The model under review builds one solid part; all positions refer to its coordinate system, in mm. Face numbers are marked on the shaded views. A direction names the side the tool comes from. Give positions to 0.01 mm unless a question says otherwise; leave off trailing zeros. Loops run counter-clockwise (first coordinate to the right, second up) from the corner with the lowest first, then second, coordinate; pieces in that order, holes last. Notation, with made-up numbers: (23, 54.5) -> (38, 54.5) arc R21 cw to (38, 88.5) -> close; hole circle Ø4 at (12, 70). An arc over 180 degrees is marked (long way). Write each question's results on one line, items separated by ' | '. Start each with the question number.
Q1. Mouldability with a two-part tool opening along Y and no side actions: class the marked faces 1, 2 and 3 as released by +Y, released by -Y, zero draft, split by the parting line, or undercut.
Q2. Wall thickness on L1, parallel to X at y = 2.95, z = 108.5; L2, parallel to X at y = 3, z = 120; L3, parallel to Y at x = 35, z = 66: over which ranges is each line inside the solid? List them lowest first. Write a range as [from, to].
Q3. Insertion check: pin 1 Ø4 at (x, z) = (27.5, 82) entering from +Y; pin 2 Ø2.5 at (y, z) = (3.5, 99) entering from -X; pin 3 Ø1.5 at (y, z) = (1.5, 98.5) entering from +X. Each pin has a flat end and moves straight along its axis. Give the tip position at first contact, or say it passes through.
Q4. We need section C-C (x = 3.5). Write out the cut boundary in (y, z), plus the area to 3 significant figures.
Q5. We need section B-B (y = 17.5). Write out the cut boundary in (x, z).
Q6. Machinability: for the marked faces 4 and 5, which of the approach directions +Z, -Z, +X, -X, +Y, -Y give a long, thin tool a straight path to every point of the face, cutting with its end or side? Answer none if there is none.
Q7. We need section A-A (z = -42). Write out the cut boundary in (x, y), plus the area to 3 significant figures.
Q8. We need section D-D (z = 72.5). Write out the cut boundary in (x, y), plus the area to 3 significant figures.
from build123d import *

# Parameters (mm, degrees)
SCHIZZO2_W                   = 15
SCHIZZO2_H                   = 5
SCHIZZO5_W                   = 15
SCHIZZO5_H                   = 5
SCHIZZO9_R                   = 3
SCHIZZO9_R_2                 = 4
ESTRUSIONE_ESTRUSIONE1_DEPTH = 5
SCHIZZO10_R                  = 3
TAGLIO_ESTRUSIONE1_DEPTH     = 144.674980425


with BuildPart() as part:
    # Sweep1: sweep along a path in Schizzo1
    with BuildLine(Plane.ZY) as sweep1_path:
        Line((0, 0), (-80, 0))
        ThreePointArc((-80, 0), (-97.5, 17.5), (-80, 35))
        Line((-80, 35), (-20, 35))
        ThreePointArc((-20, 35), (-4.629573851, 25.866600265), (-5.303061543, 8))
    # Schizzo2 → Sweep1 (sweep)
    with BuildSketch(Plane(origin=(0, 0, 0), x_dir=(-1, 0, 0), z_dir=(0, 0, -1))):
        with Locations((0, 2.5)):
            Rectangle(SCHIZZO2_W, SCHIZZO2_H)
    sweep(path=sweep1_path.line)

    # Sweep2: sweep along a path in Schizzo3
    with BuildLine(Plane.XZ) as sweep2_path:
        ThreePointArc((42.5, 96.5), (37.98987096, 70.837222968), (25, 48.25))
        ThreePointArc((25, 48.25), (12.01012904, 25.662777032), (7.5, 0))
    # Schizzo5 → Sweep2 (sweep)
    with BuildSketch(Plane.XY):
        with Locations((0, 2.5)):
            Rectangle(SCHIZZO5_W, SCHIZZO5_H)
    sweep(path=sweep2_path.line)

    # Schizzo9 → Estrusione-Estrusione1 (add)
    with BuildSketch(Plane.XZ):
        with BuildLine():
            Line((25, 96.5), (45, 96.5))
            Line((45, 96.5), (45, 102.126136458))
            ThreePointArc((45, 102.126136458), (49.5, 109), (45, 115.873863542))
            Line((45, 115.873863542), (45, 121.5))
            ThreePointArc((45, 121.5), (35, 131.5), (25, 121.5))
            Line((25, 121.5), (25, 115.873863542))
            ThreePointArc((25, 115.873863542), (20.5, 109), (25, 102.126136458))
            Line((25, 102.126136458), (25, 96.5))
        make_face()
        with Locations(Location((35, 120.5, 0), (0, 0, 270))):
            Circle(SCHIZZO9_R, mode=Mode.SUBTRACT)
        with Locations(Location((35, 108.5, 0), (0, 0, 270))):
            Circle(SCHIZZO9_R_2, mode=Mode.SUBTRACT)
    extrude(amount=-ESTRUSIONE_ESTRUSIONE1_DEPTH)

    # Schizzo10 → Taglio-Estrusione1 (cut, through all)
    with BuildSketch(Plane(origin=(0, 5, 0), x_dir=(1, 0, 0), z_dir=(0, 1, 0))):
        with Locations(Location((35, -96.5, 0), (0, 0, 270))):
            Circle(SCHIZZO10_R)
    extrude(amount=-TAGLIO_ESTRUSIONE1_DEPTH, mode=Mode.SUBTRACT)


solid = part.part
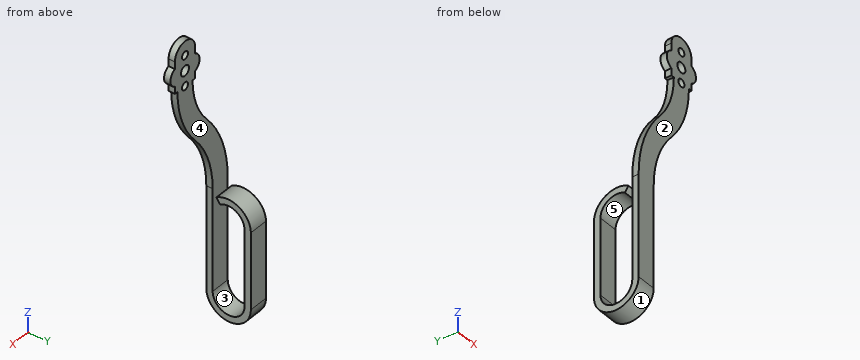
Output:
1) face 1: split by the parting line | face 2: released by -Y | face 3: undercut
2) L1: [20.52, 31], [39, 49.48] | L2: [25, 32.04], [37.96, 45] | L3: [0, 5]
3) pin 1: y = 5 | pin 2: x = 25 | pin 3: x = 45
4) outline: (0, -80) arc R17.5 ccw to (35, -80) -> (35, -20) arc R17.5 ccw to (8, -5.3) -> (10.71, -9.5) arc R12.5 cw to (30, -20) -> (30, -80) arc R12.5 cw to (5, -80) -> (5, 43.18) -> (0, 43.18) -> close | area: 1,310 mm2
5) outline: (-7.5, -97.5) -> (7.5, -97.5) -> (7.5, -92.5) -> (-7.5, -92.5) -> close; (-7.5, -7.5) -> (7.5, -7.5) -> (7.5, -2.5) -> (-7.5, -2.5) -> close
6) face 4: +Z, +X, -X | face 5: +X, -X
7) outline: (-7.5, 0) -> (7.5, 0) -> (7.5, 5) -> (-7.5, 5) -> close; (-7.5, 30) -> (7.5, 30) -> (7.5, 35) -> (-7.5, 35) -> close | area: 150 mm2
8) outline: (22.52, 0) -> (38.57, 0) -> (38.57, 5) -> (22.52, 5) -> close | area: 80.3 mm2
